Could you check a few things on this model? Use its own coordinates, in mm. A direction names the side the tool comes from. Give positions to 0.01 mm unless a question says otherwise; leave off trailing zeros. Order: outer loops, then holes, each group sorted by start corner. A loop starts at its lowest first (then second) coordinate and runs counter-clockwise, first axis right, second up. Notation, with made-up numbers: M 40.25,9.5 L 56.25,9.5 A19 ccw 56.25,26.5 Z; hole C 19,52.5 d6. An arc over 180 degrees is marked long. Use a Markdown table: item, result. Add a question column.
Item 1: Suppose I cut it at C-C on y = -26. Write out the boundary of the cut face in (x, z), plus the area to 3 significant figures.
Item 2: For faces 4 (the face through (5, 61, -6)), 5 (the face through (5, -62, -6)), 6 (the face through (5, -32, 0)), 7 (the face through (4.93, 103.03, 0.95)), 8 (the face through (5, 75, 6)), which set-ups out of +Z, -Z, +X, -X, +Y, -Y let a thin tool reach every point of the face, with its end or its side?
Item 3: If we mould it in two halves opening along Y, with no side actions, what happens to faces 1 (the face through (10, -0.5, -14.4)), 2 (the face through (4.93, -96.97, 0.95)), 3 (the face through (5, -106, 0))? For each: released by +Y, released by -Y, zero draft, split by the parting line, or undercut.
Item 4: Suppose I cut it at B-B on y = -80.5. Write out the boundary of the cut face in (x, z).
Item 5: If I drill on L1, parallel to Z at x = 2.5, y = 100 (3 decimals); L2, parallel to Y at x = 5, z = -2; L3, parallel to X at y = -40, z = -3.15, over which ranges is the centre line in solid material (lowest first)? Write a range as from..to.
Item 6: I'm going to push flat-ended pins straight in: pin 1 Ø1 at (x, z) = (6, -3.5) entering from -Y; pin 2 Ø2.5 at (x, y) = (5, -40) entering from +Z; pin 3 Ø5 at (x, z) = (9, -7) entering from -Y; pin 4 Ø3 at (x, z) = (3, -8) entering from -Y. Where does each tip first touch, or does it pass through?
Item 7: Suppose I cut it at A-A on x = 5. Write out the boundary of the cut face in (y, z) (3 decimals), plus the area to 3 significant figures.
from build123d import *

# Parameters (mm, degrees)
F0_R     = 3.175
F1_DEPTH = 10
F2_R     = 1.5
F3_DEPTH = 25


with BuildPart() as f1:
    # F0 (on Right) → F1 (new body)
    with BuildSketch(Plane.YZ):
        with BuildLine():
            Line((0, -23.9), (0, -13.9))
            ThreePointArc((0, -13.9), (-9.828784, -9.828784), (-13.9, 0))
            Line((-13.9, 0), (-50, 0))
            Line((-50, 0), (-50, 6))
            Line((-50, 6), (-100, 6))
            ThreePointArc((-100, 6), (-106, 0), (-100, -6))
            Line((-100, -6), (-23.134606, -6))
            ThreePointArc((-23.134606, -6), (-14.625491, -18.902513), (0, -23.9))
        make_face()
        with Locations((-100, 0)):
            Circle(F0_R, mode=Mode.SUBTRACT)
        with BuildLine():
            ThreePointArc((13.9, 0), (9.828784, -9.828784), (0, -13.9))
            Line((0, -13.9), (0, -23.9))
            ThreePointArc((0, -23.9), (14.625491, -18.902513), (23.134606, -6))
            Line((23.134606, -6), (100, -6))
            ThreePointArc((100, -6), (106, 0), (100, 6))
            Line((100, 6), (50, 6))
            Line((50, 6), (50, 0))
            Line((50, 0), (13.9, 0))
        make_face()
        with Locations((100, 0)):
            Circle(F0_R, mode=Mode.SUBTRACT)
    extrude(amount=F1_DEPTH)

    # F2 (on face) → F3 (cut)
    with BuildSketch(Plane(origin=(0, 0, -6), x_dir=(1, 0, 0), z_dir=(0, 0, -1))):
        with Locations((5, 40)):
            Circle(F2_R)
        with Locations((5, -40)):
            Circle(F2_R)
    extrude(amount=-F3_DEPTH, mode=Mode.SUBTRACT)


solid = f1.part
Findings below:
| question | item | result |
|---|---|---|
| 1 | outline | M 0,-6 L 10,-6 L 10,0 L 0,0 Z |
| 1 | area | 60.0 mm^2 |
| 2 | face 4 | -Z, +X, -X, +Y |
| 2 | face 5 | -Z, +X, -X, -Y |
| 2 | face 6 | +Z, +X, -X |
| 2 | face 7 | +X, -X |
| 2 | face 8 | +Z, +X, -X, +Y, -Y |
| 3 | face 1 | zero draft |
| 3 | face 2 | undercut |
| 3 | face 3 | released by -Y |
| 4 | outline | M 0,-6 L 10,-6 L 10,6 L 0,6 Z |
| 5 | L1 | z = -6..-3.175, 3.175..6 |
| 5 | L2 | y = -105.66..-102.47, -97.53..-41.5, -38.5..-13.76, 13.76..38.5, 41.5..97.53, 102.47..105.66 |
| 5 | L3 | x = 0..3.5, 6.5..10 |
| 6 | pin 1 | stops at y = -105.2 |
| 6 | pin 2 | passes through |
| 6 | pin 3 | stops at y = -103.97 |
| 6 | pin 4 | stops at y = -23 |
| 7 | outline | M -100,-6 L -41.5,-6 L -41.5,0 L -50,0 L -50,6 L -100,6 A6 ccw Z; M -38.5,-6 L -23.135,-6 A23.9 ccw 0,-23.9 A23.9 ccw 23.135,-6 L 38.5,-6 L 38.5,0 L 13.9,0 A13.9 cw 0,-13.9 A13.9 cw -13.9,0 L -38.5,0 Z; M 41.5,-6 L 100,-6 A6 ccw 100,6 L 50,6 L 50,0 L 41.5,0 Z; hole C -100,0 d6.35; hole C 100,0 d6.35 |
| 7 | area | 2,120 mm^2 |
